Can you work these out from the model? Positions are in its coordinate system, mm. A direction names the side the tool comes from. Give positions to 0.01 mm unless a question says otherwise; leave off trailing zeros. Order: outer loops, then holes, each group sorted by start corner. A loop starts at its lowest first (then second) coordinate and runs counter-clockwise, first axis right, second up. Notation, with made-up numbers: (-0.5, 23) - (11.5, 23) arc R27 cw to (11.5, 61) - close; hole circle Ø3 at (-17, 56). An arc over 180 degrees is marked (long way). Answer as CSV lines item,"result".
```python
from build123d import *

# Parameters (mm, degrees)
F0_R     = 12.831842
F0_R_2   = 11.545421
F1_DEPTH = 6.35
F2_R     = 11.571254
F2_R_2   = 6.76949
F3_DEPTH = 5.842
F4_R     = 6.77814
F4_R_2   = 4.597615
F5_DEPTH = 6.35


with BuildPart() as f1:
    # F0 (on Front) → F1 (new body)
    with BuildSketch(Plane.XZ):
        Circle(F0_R)
        Circle(F0_R_2, mode=Mode.SUBTRACT)
    extrude(amount=F1_DEPTH)

    # F2 (on Front) → F3 (join)
    with BuildSketch(Plane.XZ):
        Circle(F2_R)
        Circle(F2_R_2, mode=Mode.SUBTRACT)
    extrude(amount=F3_DEPTH)

    # F4 (on Front) → F5 (join)
    with BuildSketch(Plane.XZ):
        Circle(F4_R)
        Circle(F4_R_2, mode=Mode.SUBTRACT)
    extrude(amount=F5_DEPTH)


solid = f1.part
```
1) If we mould it in two halves opening along Z, with no side actions, what happens to faces 1 (the flat face through (6, 0, 0)), 2 (the cylindrical face through (-11.534, -6.092, 0.508)), 3 (the cylindrical face through (12.24, -3.13, 3.85))? For each: +Z half, -Z half, draft (parallel to the pull), parting line (faces both ways), or undercut.
Answer block:
face 1,"draft"
face 2,"undercut"
face 3,"parting line"
2) I want a section at B-B on z = 0. Write out the boundary of the cut face in (x, y).
Answer block:
outline,"(-12.83, -6.35) - (-11.55, -6.35) - (-11.55, -5.84) - (-6.78, -5.84) - (-6.78, -6.35) - (-4.6, -6.35) - (-4.6, 0) - (-12.83, 0) - close; (4.6, -6.35) - (6.78, -6.35) - (6.78, -5.84) - (11.55, -5.84) - (11.55, -6.35) - (12.83, -6.35) - (12.83, 0) - (4.6, 0) - close"
3) I want a section at D-D on z = -8.75. Write out the boundary of the cut face in (x, y), plus the area to 3 significant figures.
Answer block:
outline,"(-9.39, -6.35) - (-7.53, -6.35) - (-7.53, -5.84) - (7.53, -5.84) - (7.53, -6.35) - (9.39, -6.35) - (9.39, 0) - (-9.39, 0) - close"
area,"112 mm2"
4) Which directions (+Z, -Z, +X, -X, +Y, -Y) give clear straight access to the entire face, cutting with the end or side of a thin tool? Please do faces 4 (the cylindrical face through (4.385, -3.131, 1.381)), 5 (the cylindrical face through (3.64, -6.09, 5.72)).
Answer block:
face 4,"+Y, -Y"
face 5,"-Y"
5) I'm going to push a flat-ended pin straight in: P1, Ø1, axis at y = -5, z = -5, coming from the -X side. Where does the tip first touch, or does it pass through?
Answer block:
P1,"x = -12.02"
6) I want a section at C-C on y = -4.75. Write out the boundary of the cut face in (x, z).
Answer block:
outline,"circle Ø25.66 at (0, 0); hole circle Ø9.2 at (0, 0)"
7) I need wall thicknesses on line 1 along Z through (x, y) = (0, -6.05); line 2 along X through (y, z) = (-6, -4.25); line 3 along Z through (x, y) = (0, -1.5). Which ranges of each line are inside material? Lowest first, please. Write a range as [from, to].
Answer block:
line 1,"[-12.83, -11.55], [-6.78, -4.6], [4.6, 6.78], [11.55, 12.83]"
line 2,"[-12.11, -10.73], [-5.28, -1.75], [1.75, 5.28], [10.73, 12.11]"
line 3,"[-12.83, -4.6], [4.6, 12.83]"
8) I want a section at A-A on x = 0. Write out the boundary of the cut face in (y, z), plus the area to 3 significant figures.
Answer block:
outline,"(-6.35, -12.83) - (0, -12.83) - (0, -4.6) - (-6.35, -4.6) - (-6.35, -6.78) - (-5.84, -6.78) - (-5.84, -11.55) - (-6.35, -11.55) - close; (-6.35, 4.6) - (0, 4.6) - (0, 12.83) - (-6.35, 12.83) - (-6.35, 11.55) - (-5.84, 11.55) - (-5.84, 6.78) - (-6.35, 6.78) - close"
area,"99.7 mm2"
